Part print with two shaded views. Sizes in mm from the minimum x, y, z corner. Give positions to 0.01 mm unless a question says otherwise; leave off trailing zeros. Write each loop counter-clockwise with the first axis right and the second up, starting at its lowest first coordinate (ties: lowest second). Pieces come first, ordered by that corner, then holes.
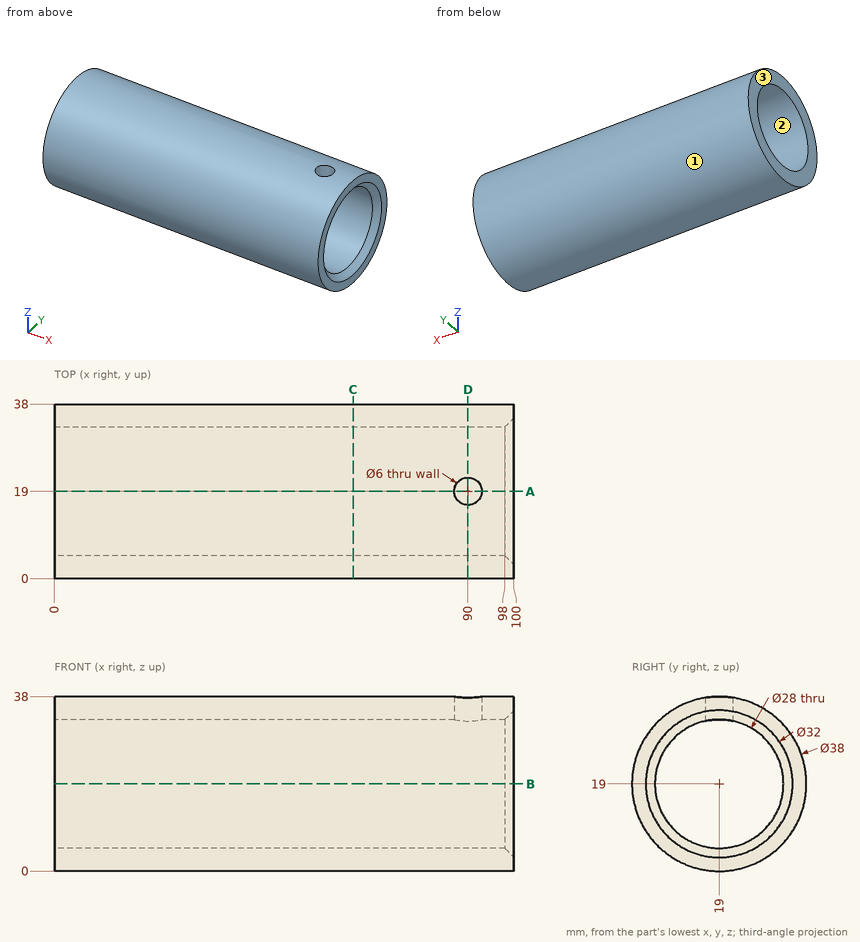
1) Flat gauge pins, fed straight in: P1, Ø7, axis at x = 90, y = 19, coming from the -Z side; P2, Ø1, axis at x = 79.5, y = 28.5, coming from the +Z side; P3, Ø3, axis at x = 45, z = 6.5, coming from the -Y side. Where does each tip first touch, or does it go through?
Check result:
P1: stops at z = 0
P2: stops at z = 35.73
P3: stops at y = 3.51
2) Saw through at C-C (x = 65). Write the cut outline in (y, z).
Check result:
outline: circle Ø38 at (19, 19); hole circle Ø28 at (19, 19)
3) Saw through at B-B (z = 19). Write the cut outline in (x, y).
Check result:
outline: (0, 0) - (100, 0) - (100, 3) - (98, 5) - (0, 5) - close; (0, 33) - (98, 33) - (100, 35) - (100, 38) - (0, 38) - close
4) Drill centre lines: L1, parallel to Z at x = 66, y = 19; L2, parallel to Z at x = 13, y = 30.5; L3, parallel to Y at x = 43, z = 11. Where is each one in solid material? Low to high.
Check result:
L1: z = 0 to 5, 33 to 38
L2: z = 3.88 to 11.02, 26.98 to 34.12
L3: y = 1.77 to 7.51, 30.49 to 36.23
5) Saw through at A-A (y = 19). Write the cut outline in (x, z), and give its area (3 significant figures).
Check result:
outline: (0, 0) - (100, 0) - (100, 3) - (98, 5) - (0, 5) - close; (0, 33) - (87, 33) - (87, 38) - (0, 38) - close; (93, 33) - (98, 33) - (100, 35) - (100, 38) - (93, 38) - close
area: 966 mm2
6) Saw through at D-D (x = 90). Write the cut outline in (y, z), and give its area (3 significant figures).
Check result:
outline: (16, 32.67) - (16, 37.76) arc R19 ccw (long way) to (22, 37.76) - (22, 32.67) arc R14 cw (long way) to start
area: 488 mm2
7) Mould opens along Z. For the marked faces 1, 2 and 3 say: +Z half, -Z half, draft (parallel to the pull), parting line (faces both ways), or undercut.
Check result:
face 1: parting line
face 2: undercut
face 3: draft
